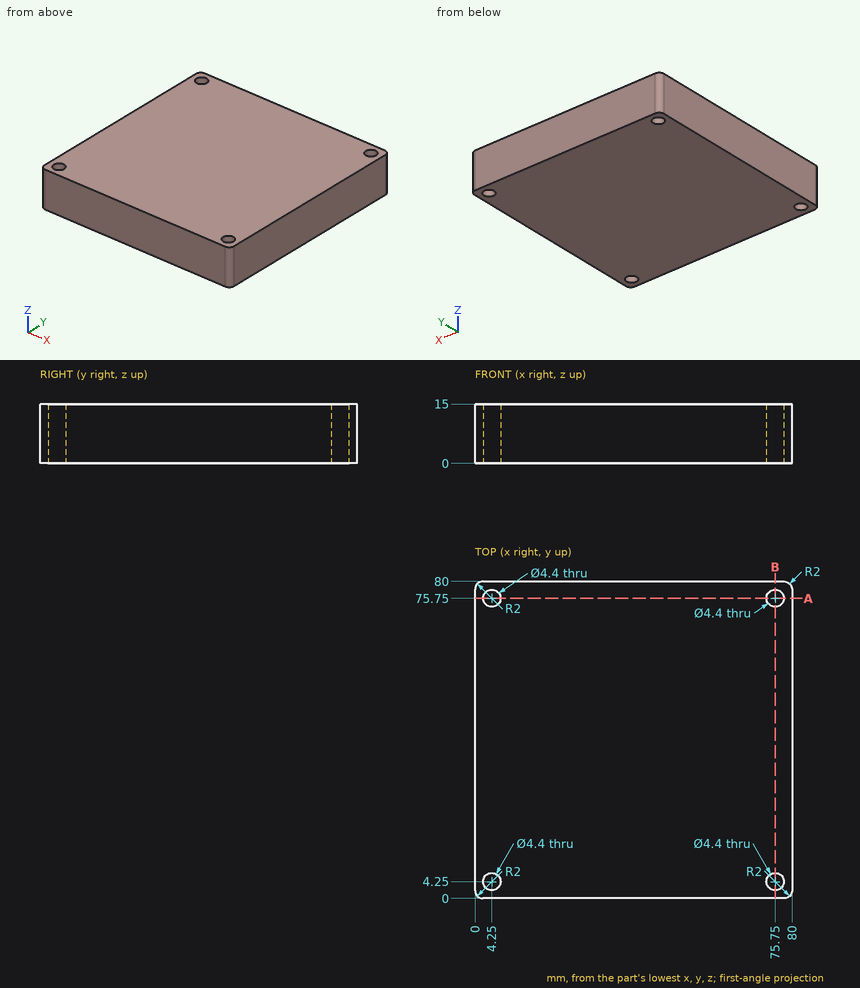
Here's the drawing with two shaded views (mm, measured from the low corner). I have some questions. Give positions to 0.01 mm unless a question says otherwise; leave off trailing zeros. Write each loop counter-clockwise with the first axis right and the second up, starting at its lowest first coordinate (ties: lowest second). Pieces come first, ordered by that corner, then holes. Notation, with made-up numbers: (65, 7.25) -> (77, 7.25) arc R10 ccw to (77, 13.25) -> close; hole circle Ø1 at (7.25, 77.5). An arc over 180 degrees is marked (long way). One line per item, written item: value.
Q1. Please list where these lines run through material, in increasing order: line 1 (Y direction, x = 75.75, z = 7.25); line 2 (X direction, y = 77, z = 10.25). Write a range as [from, to].
Results found:
line 1: y = [0, 2.05], [6.45, 73.55], [77.95, 80]
line 2: x = [0, 2.44], [6.06, 73.94], [77.56, 80]
Q2. Imagine slicing it at A-A on y = 75.75. Please give me the cut outline in (x, z).
Results found:
outline: (0, 0) -> (2.05, 0) -> (2.05, 15) -> (0, 15) -> close; (6.45, 0) -> (73.55, 0) -> (73.55, 15) -> (6.45, 15) -> close; (77.95, 0) -> (80, 0) -> (80, 15) -> (77.95, 15) -> close
